Read the model definition and answer for the solid it produces. Units are mm, in the model's axes. A direction names the side the tool comes from. Coordinates: 2 decimals unless noted, no trailing zeros. Order: outer loops, then holes, each group sorted by start corner. A loop starts at its lowest first (then second) coordinate and runs counter-clockwise, first axis right, second up. Notation, with made-up numbers: M 16,72 L 40,72 A25 ccw 40,105 Z; hole C 68,37 d1. An arc over 180 degrees is marked long. One line per question, with ' | ' between items. Start each with the question number.
1) Find section C-C, the plane z = 2.75. Write down the section's boundary in (x, y), plus the area to 3 significant figures.
2) Find section D-D, the plane x = 20.5. Write down the section's boundary in (y, z), plus the area to 3 significant figures.
3) The mould has two halves that part along Y. Classify faces 4 (the face through (28, 0, 5)), 5 (the face through (0, 8, 5)), 6 (the face through (16, 0, 10)): +Y half, -Y half, draft (parallel to the pull), parting line (faces both ways), or undercut.
4) Find section A-A, the plane x = 9. Write down the section's boundary in (y, z).
5) Consider probe 1 along Y at (x, z) = (-3.5, 3); probe 2 along X at (y, z) = (4, 6.5); probe 3 along Y at (x, z) = (-21, 5). Determine where each line is inside the solid, lowest interval first.
6) Find section B-B, the plane y = 0. Write down the section's boundary in (x, z).
7) A tool of negligible diameter and unlimited length cuts with its end or side. For faces 1 (the face through (12, 0.1, 12.5)), 2 (the face through (0, 5, 0)), 3 (the face through (20, 4, 5)), from which of +Z, -Z, +X, -X, +Y, -Y can it reach the whole face along a straight path? Write none if from no direction.
8) Given P1, Ø5, axis at x = -18, y = 0.5, coming from the -Z side; P2, Ø1.1, axis at y = -0.5, z = 12.5, coming from the +X side; P3, Ø3.5, axis at x = 20, y = 0, coming from the +Z side, each flat-ended and moving along its own axis, determine where each tip first touches the part or whether it passes through.
from build123d import *

# Parameters (mm, degrees)
F0_R     = 3
F1_DEPTH = 13
F2_W     = 40
F2_H     = 9
F3_DEPTH = 10
F4_R     = 2


with BuildPart() as f1:
    # F0 (on Top) → F1 (new body)
    with BuildSketch(Plane.XY):
        Polygon((-28, -8), (28, -8), (28, 0), (28, 8), (0, 8), (-28, 8), (-28, 0), align=None)
        with BuildLine():
            ThreePointArc((-17, 0), (-20, -3), (-23, 0))
            ThreePointArc((-23, 0), (-20, 3), (-17, 0))
        make_face(mode=Mode.SUBTRACT)
        Polygon((-12, 4.5), (0, 4.5), (12, 4.5), (12, -4.5), (-12, -4.5), align=None, mode=Mode.SUBTRACT)
        with Locations((20, 0)):
            Circle(F0_R, mode=Mode.SUBTRACT)
    extrude(amount=F1_DEPTH)

    # F2 (on face) → F3 (cut)
    with BuildSketch(Plane(origin=(0, 0, 0), x_dir=(1, 0, 0), z_dir=(0, 0, -1))):
        Rectangle(F2_W, F2_H)
    extrude(amount=-F3_DEPTH, mode=Mode.SUBTRACT)

    # F4
    f4_edges = [f1.edges().sort_by_distance(p)[0] for p in [
        (-28, -8, 6.5),
        (0, -8, 13),
        (0, 8, 13),
        (-28, 8, 6.5),
        (-28, 0, 13),
        (28, 8, 6.5),
        (28, 0, 13),
        (28, -8, 6.5),
        (-12, 0, 10),
        (12, 0, 10),
    ]]
    fillet(f4_edges, radius=F4_R)


solid = f1.part
Report:
1) outline: M -28,-6 A2 ccw -26,-8 L 26,-8 A2 ccw 28,-6 L 28,6 A2 ccw 26,8 L -26,8 A2 ccw -28,6 Z; hole M -20,-4.5 L 20,-4.5 L 20,-3 A3 ccw 20,3 L 20,4.5 L -20,4.5 L -20,3 A3 ccw -20,-3 Z | area: 504 mm^2
2) outline: M -8,0 L -2.96,0 L -2.96,13 L -6,13 A2 ccw -8,11 Z; M 2.96,0 L 8,0 L 8,11 A2 ccw 6,13 L 2.96,13 Z | area: 129 mm^2
3) face 4: draft | face 5: +Y half | face 6: undercut
4) outline: M -8,0 L -4.5,0 L -4.5,13 L -6,13 A2 ccw -8,11 Z; M 4.5,0 L 8,0 L 8,11 A2 ccw 6,13 L 4.5,13 Z
5) probe 1: y = -8 to -4.5, 4.5 to 8 | probe 2: x = -28 to -20, 20 to 28 | probe 3: y = -8 to -2.83, 2.83 to 8
6) outline: M -28,0 L -23,0 L -23,13 L -26,13 A2 ccw -28,11 Z; M -17,10 L -14,10 A2 ccw -12,12 L -12,13 L -17,13 Z; M 12,12 A2 ccw 14,10 L 17,10 L 17,13 L 12,13 Z; M 23,0 L 28,0 L 28,11 A2 ccw 26,13 L 23,13 Z
7) face 1: +Z, -Z | face 2: -Z, +X, -X, +Y, -Y | face 3: -Z
8) P1: stops at z = 10 | P2: stops at x = 27.76 | P3: passes through
